CAD build for the part. Positions are in the model's coordinates, mm. A direction names the side the tool comes from. Coordinates: 2 decimals unless noted, no trailing zeros. Loops run counter-clockwise (first coordinate to the right, second up) from the corner with the lowest first, then second, coordinate; pieces in that order, holes last. Notation, with made-up numbers: (8.25, 80) - (61.25, 80) arc R11 cw to (61.25, 100) - close; hole circle Ø6 at (-13, 19). An arc over 180 degrees is marked (long way). Put each result on its own line as item: value.
```python
from build123d import *

# Parameters (mm, degrees)
SKETCH1_W                        = 38.1
SKETCH1_H                        = 292.1
BASE_FLANGE1_DEPTH               = 0.508
SKETCHED_START                   = -19.05
SKETCHED_BEND5_DEPTH             = 38.1
SKETCHED_BEND5_2_DEPTH           = 38.1
SKETCHED_BEND8_DEPTH             = 38.1
SKETCHED_BEND8_2_DEPTH           = 38.1
F_1_4_0_25_DIAMETER_HOLE4_D      = 6.35
F_1_4_0_25_DIAMETER_HOLE4_DEPTH  = 0.508
F_1_8_0_125_DIAMETER_HOLE1_D     = 3.175
F_1_8_0_125_DIAMETER_HOLE1_DEPTH = 0.508


# Read off the part's stored shape, not the designer's step: Sketched Bend5, Sketched Bend8
# Sheet-metal steps are written as plain solids
with BuildPart() as part:
    # Sketch1 → Base-Flange1 (new body)
    with BuildSketch(Plane.XY):
        Rectangle(SKETCH1_W, SKETCH1_H)
    extrude(amount=-BASE_FLANGE1_DEPTH)

    # Sketched Bend5 outline → Sketched Bend5 (cut)
    with BuildSketch(Plane.YZ.offset(SKETCHED_START)):
        with BuildLine():
            Line((146.05, 0), (108.175204196, 0))
            ThreePointArc((108.175204196, 0), (107.734237547, -0.373760644), (107.171984579, -0.508))
            Line((107.171984579, -0.508), (146.05, -0.508))
            Line((146.05, -0.508), (146.05, 0))
        make_face()
    extrude(amount=SKETCHED_BEND5_DEPTH, mode=Mode.SUBTRACT)

    # Sketched Bend5 2 outline → Sketched Bend5 2 (add)
    with BuildSketch(Plane.YZ.offset(SKETCHED_START)):
        with BuildLine():
            ThreePointArc((108.175204196, 0), (108.354701007, 0.349029345), (108.416584579, 0.7366))
            Line((108.416584579, 0.7366), (108.416584579, 38.058584579))
            Line((108.416584579, 38.058584579), (107.908584579, 38.058584579))
            Line((107.908584579, 38.058584579), (107.908584579, 0.7366))
            ThreePointArc((107.908584579, 0.7366), (107.692839434, 0.215745145), (107.171984579, 0))
            Line((107.171984579, 0), (108.175204196, 0))
        make_face()
    extrude(amount=SKETCHED_BEND5_2_DEPTH)

    # Sketched Bend8 outline → Sketched Bend8 (cut)
    with BuildSketch(Plane.YZ.offset(SKETCHED_START)):
        with BuildLine():
            ThreePointArc((-107.171984579, -0.508), (-107.734237547, -0.373760644), (-108.175204196, 0))
            Line((-108.175204196, 0), (-146.05, 0))
            Line((-146.05, 0), (-146.05, -0.508))
            Line((-146.05, -0.508), (-107.171984579, -0.508))
        make_face()
    extrude(amount=SKETCHED_BEND8_DEPTH, mode=Mode.SUBTRACT)

    # Sketched Bend8 2 outline → Sketched Bend8 2 (add)
    with BuildSketch(Plane.YZ.offset(SKETCHED_START)):
        with BuildLine():
            Line((-107.908584579, 0.7366), (-107.908584579, 38.058584579))
            Line((-107.908584579, 38.058584579), (-108.416584579, 38.058584579))
            Line((-108.416584579, 38.058584579), (-108.416584579, 0.7366))
            ThreePointArc((-108.416584579, 0.7366), (-108.354701007, 0.349029345), (-108.175204196, 0))
            Line((-108.175204196, 0), (-107.171984579, 0))
            ThreePointArc((-107.171984579, 0), (-107.692839434, 0.215745145), (-107.908584579, 0.7366))
        make_face()
    extrude(amount=SKETCHED_BEND8_2_DEPTH)

    # 1/4 (0.25) Diameter Hole4
    with Locations(Plane(origin=(-3.81, 107.908584579, 7.0866), x_dir=(0, 0, -1), z_dir=(0, -1, 0))):
        with Locations((0, 0)):
            f_1_4_0_25_diameter_hole4 = Hole(F_1_4_0_25_DIAMETER_HOLE4_D / 2, depth=F_1_4_0_25_DIAMETER_HOLE4_DEPTH)

    # 1/8 (0.125) Diameter Hole1
    with Locations(Plane(origin=(-12.7, 107.908584579, 29.9466), x_dir=(0, 0, -1), z_dir=(0, -1, 0))):
        with Locations((0, 0)):
            f_1_8_0_125_diameter_hole1 = Hole(F_1_8_0_125_DIAMETER_HOLE1_D / 2, depth=F_1_8_0_125_DIAMETER_HOLE1_DEPTH)

    # Mirror1: 1/4 (0.25) Diameter Hole4, 1/8 (0.125) Diameter Hole1 across plane
    add(f_1_4_0_25_diameter_hole4.mirror(Plane.ZX), mode=Mode.SUBTRACT)
    add(f_1_8_0_125_diameter_hole1.mirror(Plane.ZX), mode=Mode.SUBTRACT)


solid = part.part
```
Q1. Pin check, flat tips, straight feed: pin 1 Ø8.5 at (x, z) = (-3.81, 7.09) entering from +Y; pin 2 Ø8 at (x, y) = (13, 20.5) entering from +Z. Stop position of each tip, or through.
Determined:
pin 1: y = 108.42
pin 2: z = 0
Q2. Slice it at D-D, the plane y = 64. Give the cut face in (x, z).
Determined:
outline: (-19.05, -0.51) - (19.05, -0.51) - (19.05, 0) - (-19.05, 0) - close
Q3. Mould opens along Z. For faces 1 (the cylindrical face through (-5.03, 108.17, 10.02)), 2 (the flat face through (0, 108.417, 19)), 3 (the flat face through (0, 2, -0.508)), 4 (the flat face through (0, 2, 0)) say: +Z half, -Z half, draft (parallel to the pull), parting line (faces both ways), or undercut.
Determined:
face 1: undercut
face 2: draft
face 3: -Z half
face 4: +Z half
Q4. Slice it at B-B, the plane z = 22.5. Give the cut face in (x, y).
Determined:
outline: (-19.05, -108.42) - (19.05, -108.42) - (19.05, -107.91) - (-19.05, -107.91) - close; (-19.05, 107.91) - (19.05, 107.91) - (19.05, 108.42) - (-19.05, 108.42) - close
Q5. Tool access for faces 5 (the flat face through (0, 107.909, 20)), 6 (the cylindrical face through (-5.03, -108.17, 10.02)): list every direction of +Z, -Z, +X, -X, +Y, -Y with a clear straight run to the whole face (end or side of a thin tool).
Determined:
face 5: +Z, +X, -X
face 6: +Y, -Y
Q6. Slice it at C-C, the plane x = 7.5. Give the cut face in (y, z).
Determined:
outline: (-108.42, 0.74) arc R1.24 ccw to (-107.17, -0.51) - (107.17, -0.51) arc R1.24 ccw to (108.42, 0.74) - (108.42, 38.06) - (107.91, 38.06) - (107.91, 0.74) arc R0.74 cw to (107.17, 0) - (-107.17, 0) arc R0.74 cw to (-107.91, 0.74) - (-107.91, 38.06) - (-108.42, 38.06) - close
Q7. Wall check: L1, parallel to Y at x = 0.5, z = 35.5; L2, parallel to Z at x = -3.81, y = -108.15; L3, parallel to Z at x = -4.5, y = -32.5. Give the ranges that are in metal, low to high. Write a range as from..to.
Determined:
L1: -108.42..-107.91, 107.91..108.42
L2: -0.03..3.91, 10.26..38.06
L3: -0.51..0
Q8. Slice it at A-A, the plane x = -3.81. Give the cut face in (y, z), then the cut area to 3 significant figures.
Determined:
outline: (-108.42, 0.74) arc R1.24 ccw to (-107.17, -0.51) - (107.17, -0.51) arc R1.24 ccw to (108.42, 0.74) - (108.42, 3.91) - (107.91, 3.91) - (107.91, 0.74) arc R0.74 cw to (107.17, 0) - (-107.17, 0) arc R0.74 cw to (-107.91, 0.74) - (-107.91, 3.91) - (-108.42, 3.91) - close; (-108.42, 10.26) - (-107.91, 10.26) - (-107.91, 38.06) - (-108.42, 38.06) - close; (107.91, 10.26) - (108.42, 10.26) - (108.42, 38.06) - (107.91, 38.06) - close
area: 142 mm2
